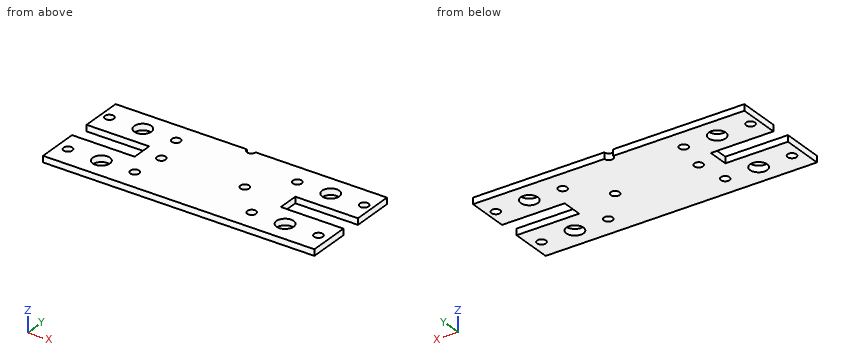
from build123d import *

# Parameters (mm, degrees)
ESQUISSE1_W             = 130
ESQUISSE1_H             = 50
ESQUISSE1_R             = 2.1
ESQUISSE1_R_2           = 4.1
BOSS_EXTRU_1_DEPTH      = 3
ENL_V_MAT_EXTRU_1_REACH = 5
ESQUISSE2_W             = 30
ESQUISSE2_H             = 10


with BuildPart() as part:
    # Esquisse1 → Boss.-Extru.1 (new body)
    with BuildSketch(Plane.XY):
        with Locations((65, 25)):
            Rectangle(ESQUISSE1_W, ESQUISSE1_H)
        with Locations((4, 40)):
            Circle(ESQUISSE1_R, mode=Mode.SUBTRACT)
        with Locations((20, 40)):
            Circle(ESQUISSE1_R_2, mode=Mode.SUBTRACT)
        with Locations((36, 40)):
            Circle(ESQUISSE1_R, mode=Mode.SUBTRACT)
        with Locations((94, 40)):
            Circle(ESQUISSE1_R, mode=Mode.SUBTRACT)
        with Locations((110, 40)):
            Circle(ESQUISSE1_R_2, mode=Mode.SUBTRACT)
        with Locations((126, 40)):
            Circle(ESQUISSE1_R, mode=Mode.SUBTRACT)
        with Locations((5, 10)):
            Circle(ESQUISSE1_R, mode=Mode.SUBTRACT)
        with Locations((21, 10)):
            Circle(ESQUISSE1_R_2, mode=Mode.SUBTRACT)
        with Locations((37, 10)):
            Circle(ESQUISSE1_R, mode=Mode.SUBTRACT)
        with Locations((93, 10)):
            Circle(ESQUISSE1_R, mode=Mode.SUBTRACT)
        with Locations((109, 10)):
            Circle(ESQUISSE1_R_2, mode=Mode.SUBTRACT)
        with Locations((125, 10)):
            Circle(ESQUISSE1_R, mode=Mode.SUBTRACT)
        with Locations((39.3, 25)):
            Circle(ESQUISSE1_R, mode=Mode.SUBTRACT)
        with Locations((79.3, 25)):
            Circle(ESQUISSE1_R, mode=Mode.SUBTRACT)
    extrude(amount=BOSS_EXTRU_1_DEPTH)

    # Esquisse2 → Enlèv. mat.-Extru.1 (cut, up to next)
    with BuildSketch(Plane(origin=(0, 0, 0), x_dir=(-1, 0, 0), z_dir=(0, 0, -1)), mode=Mode.PRIVATE) as enl_v_mat_extru_1_sk1:
        with Locations((-15, 25)):
            Rectangle(ESQUISSE2_W, ESQUISSE2_H)
    enl_v_mat_extru_1_tool1 = extrude(enl_v_mat_extru_1_sk1.sketch, amount=-ENL_V_MAT_EXTRU_1_REACH, mode=Mode.PRIVATE) & part.part
    add(enl_v_mat_extru_1_tool1.solids().sort_by_distance((15, 25, 0))[0], mode=Mode.SUBTRACT)
    # Esquisse2 → Enlèv. mat.-Extru.1 (cut, up to next)
    with BuildSketch(Plane(origin=(0, 0, 0), x_dir=(-1, 0, 0), z_dir=(0, 0, -1)), mode=Mode.PRIVATE) as enl_v_mat_extru_1_sk2:
        with Locations((-115, 25)):
            Rectangle(ESQUISSE2_W, ESQUISSE2_H)
    enl_v_mat_extru_1_tool2 = extrude(enl_v_mat_extru_1_sk2.sketch, amount=-ENL_V_MAT_EXTRU_1_REACH, mode=Mode.PRIVATE) & part.part
    add(enl_v_mat_extru_1_tool2.solids().sort_by_distance((115, 25, 0))[0], mode=Mode.SUBTRACT)
    # Esquisse2 → Enlèv. mat.-Extru.1 (cut, up to next)
    with BuildSketch(Plane(origin=(0, 0, 0), x_dir=(-1, 0, 0), z_dir=(0, 0, -1)), mode=Mode.PRIVATE) as enl_v_mat_extru_1_sk3:
        with BuildLine():
            Line((-62.9, 50), (-67.1, 50))
            ThreePointArc((-67.1, 50), (-65, 47.9), (-62.9, 50))
        make_face()
    enl_v_mat_extru_1_tool3 = extrude(enl_v_mat_extru_1_sk3.sketch, amount=-ENL_V_MAT_EXTRU_1_REACH, mode=Mode.PRIVATE) & part.part
    add(enl_v_mat_extru_1_tool3.solids().sort_by_distance((65, 49.108732, 0))[0], mode=Mode.SUBTRACT)


solid = part.part
Verification items for the finished model (mm, model axes). Give positions to 0.01 mm unless a question says otherwise; leave off trailing zeros. Loops run counter-clockwise (first coordinate to the right, second up) from the corner with the lowest first, then second, coordinate; pieces in that order, holes last. Notation, with made-up numbers: (25, 38) - (69, 38) arc R20 cw to (69, 47) - close; hole circle Ø7 at (11, -24). An arc over 180 degrees is marked (long way). Write item = value, one per line. Start each with the question number.
Q1. Cross-section at D-D, the plane x = 79.3. Enter the section's corners in (y, z), and give its area (3 significant figures).
Q2. Cross-section at B-B, the plane z = 1.65. State how many separate pieces and enclosed holes the cut face has, and give its area (3 significant figures).
Q3. Depth check by flat-ended pin: P1, Ø5, axis at x = 109, y = 10, coming from the -Z side. Enter the tip coordinate at first touch or a pass-through.
Q4. Thickness scan on line 1 (Y direction, x = 36, z = 1.65); line 2 (Y direction, x = 5, z = 0.95); line 3 (Y direction, x = 25.5, z = 0.55). Record the ranges inside material, lowest first.
Q5. Cross-section at C-C, the plane x = 21.5. Enter the section's corners in (y, z), and give its area (3 significant figures).
Q6. Cross-section at A-A, the plane x = 120. Enter the section's corners in (y, z), and give its area (3 significant figures).
Answer key:
q1.outline = (0, 0) - (22.9, 0) - (22.9, 3) - (0, 3) - close; (27.1, 0) - (50, 0) - (50, 3) - (27.1, 3) - close
q1.area = 137 mm^2
q2.separate_pieces = 1
q2.enclosed_holes = 14
q2.area = 5,540 mm^2
q3.P1 = through
q4.line_1 = 0 to 8.15, 11.85 to 37.9, 42.1 to 50
q4.line_2 = 0 to 7.9, 12.1 to 20, 30 to 38.15, 41.85 to 50
q4.line_3 = 0 to 20, 30 to 50
q5.outline = (0, 0) - (5.93, 0) - (5.93, 3) - (0, 3) - close; (14.07, 0) - (20, 0) - (20, 3) - (14.07, 3) - close; (30, 0) - (36.18, 0) - (36.18, 3) - (30, 3) - close; (43.82, 0) - (50, 0) - (50, 3) - (43.82, 3) - close
q5.area = 72.7 mm^2
q6.outline = (0, 0) - (20, 0) - (20, 3) - (0, 3) - close; (30, 0) - (50, 0) - (50, 3) - (30, 3) - close
q6.area = 120 mm^2
